from build123d import *

# Parameters (mm, degrees)
PAD_DEPTH       = 20
PAD001_DEPTH    = 10
PAD002_DEPTH    = 15
SKETCH003_R     = 2.1
POCKET_DEPTH    = 8.001
SKETCH004_R     = 3.75
POCKET001_DEPTH = 4
SKETCH005_W     = 10
SKETCH005_H     = 55
POCKET002_DEPTH = 40
SKETCH006_R     = 15
POCKET003_DEPTH = 95.001


with BuildPart() as part:
    # Sketch → Pad (new body, symmetric)
    with BuildSketch(Plane.XZ):
        Polygon((0, 163), (0, 0), (105, 0), (105, 8), (15, 8), (15, 163), align=None)
    extrude(amount=PAD_DEPTH, both=True)

    # Sketch001 (on Face8 of Pad) → Pad001 (join)
    with BuildSketch(Plane.XZ.offset(20)):
        Polygon((15, 38), (90, 8), (15, 8), align=None)
    pad001 = extrude(amount=-PAD001_DEPTH)

    # Mirrored: Pad001 across XZ
    add(pad001.mirror(Plane.XZ))

    # Sketch002 (on Face1 of Mirrored) → Pad002 (join)
    with BuildSketch(Plane(origin=(0, 0, 0), x_dir=(0, -1, 0), z_dir=(-1, 0, 0))):
        Polygon((-40, 0), (-20, 0), (-20, 163), (-30, 163), (-30, 8), (-40, 8), align=None)
    pad002 = extrude(amount=-PAD002_DEPTH)

    # Mirrored001: Pad002 across Sketch002 V_Axis
    add(pad002.mirror(Plane(origin=(0, 0, 0), x_dir=(-1, 0, 0), z_dir=(0, -1, 0))))

    # Sketch003 (on Face11 of Mirrored001) → Pocket (cut, through all)
    with BuildSketch(Plane.XY.offset(8)):
        with Locations((7.5, 35)):
            Circle(SKETCH003_R)
        with Locations((7.5, -35)):
            Circle(SKETCH003_R)
        with Locations((97, 15.5)):
            Circle(SKETCH003_R)
        with Locations((97, -15.5)):
            Circle(SKETCH003_R)
    extrude(amount=-POCKET_DEPTH, mode=Mode.SUBTRACT)

    # Sketch004 (on Face15 of Pocket) → Pocket001 (cut)
    with BuildSketch(Plane.XY.offset(8)):
        with Locations((7.5, 35)):
            Circle(SKETCH004_R)
        with Locations((97, 15.5)):
            Circle(SKETCH004_R)
        with Locations((97, -15.5)):
            Circle(SKETCH004_R)
        with Locations((7.5, -35)):
            Circle(SKETCH004_R)
    extrude(amount=-POCKET001_DEPTH, mode=Mode.SUBTRACT)

    # Sketch005 (on Face12 of Pocket001) → Pocket002 (cut)
    with BuildSketch(Plane.XZ.offset(20)):
        with Locations((5, 135.5)):
            Rectangle(SKETCH005_W, SKETCH005_H)
    extrude(amount=-POCKET002_DEPTH, mode=Mode.SUBTRACT)

    # Sketch006 (on Face23 of Pocket002) → Pocket003 (cut, through all)
    with BuildSketch(Plane(origin=(10, 0, 0), x_dir=(0, -1, 0), z_dir=(-1, 0, 0))):
        with Locations((0, 141)):
            Circle(SKETCH006_R)
    extrude(amount=-POCKET003_DEPTH, mode=Mode.SUBTRACT)


solid = part.part
Read the model definition and answer for the solid it produces. Units are mm, in the model's axes. A direction names the side the tool comes from. Round coordinates to 2 decimals unless told otherwise and drop trailing zeros. Write each loop counter-clockwise with the first axis right and the second up, starting at its lowest first coordinate (ties: lowest second). Pieces come first, ordered by that corner, then holes. Notation, with made-up numbers: (69.5, -38.5) - (112.5, -38.5) arc R29 cw to (112.5, -2.5) - close; hole circle Ø11 at (76.5, 71). An arc over 180 degrees is marked (long way). Use a Markdown table: item, result.
(1) The part is cut by section A-A (x = 7.5). Write down the section's boundary in (y, z), then the cut area to 3 significant figures.
Reported:
| item | result |
|---|---|
| outline | (-40, 0) - (-37.1, 0) - (-37.1, 4) - (-38.75, 4) - (-38.75, 8) - (-40, 8) - close; (-32.9, 0) - (32.9, 0) - (32.9, 4) - (31.25, 4) - (31.25, 8) - (30, 8) - (30, 163) - (20, 163) - (20, 108) - (-20, 108) - (-20, 163) - (-30, 163) - (-30, 8) - (-31.25, 8) - (-31.25, 4) - (-32.9, 4) - close; (37.1, 0) - (40, 0) - (40, 8) - (38.75, 8) - (38.75, 4) - (37.1, 4) - close |
| area | 7,650 mm2 |
(2) Straight lines are drawn through the part: line 1 along Y through (x, z) = (97, 2.7); line 2 along Y through (x, z) = (7.5, 2.8); line 3 along X through (y, z) = (15, 5). For each, find the intervals that lie inside material, in ascending order. Write a range as [from, to].
Reported:
| item | result |
|---|---|
| line 1 | [-20, -17.6], [-13.4, 13.4], [17.6, 20] |
| line 2 | [-40, -37.1], [-32.9, 32.9], [37.1, 40] |
| line 3 | [0, 93.28], [100.72, 105] |
(3) The part is cut by section B-B (y = 35). Write down the section's boundary in (x, z).
Reported:
| item | result |
|---|---|
| outline | (0, 0) - (5.4, 0) - (5.4, 4) - (3.75, 4) - (3.75, 8) - (0, 8) - close; (9.6, 0) - (15, 0) - (15, 8) - (11.25, 8) - (11.25, 4) - (9.6, 4) - close |
(4) Which of the six approach directions +Z, -Z, +X, -X, +Y, -Y give full straight-line access (tool end or side, diameter ignored) to faces 1 (the cylindrical face through (10.964, -36.436, 6.028)), 2 (the flat face through (7, 30, 87)), 3 (the flat face through (51, -20, 11)), 4 (the flat face through (7, -30, 87)), 5 (the flat face through (5, -20, 136))?
Reported:
| item | result |
|---|---|
| face 1 | +Z |
| face 2 | +Z, +X, -X, +Y |
| face 3 | +Z, -Z, +X, -Y |
| face 4 | +Z, +X, -X, -Y |
| face 5 | +Z, -X |
(5) The mould has two halves that part along Y. Classify faces 6 (the flat face through (7, -40, 4)), 7 (the cylindrical face through (94.9, -15.41, 2.03)), 8 (the flat face through (105, 0, 4)): released by +Y, released by -Y, zero draft, split by the parting line, or undercut.
Reported:
| item | result |
|---|---|
| face 6 | released by -Y |
| face 7 | undercut |
| face 8 | zero draft |
(6) The part is cut by section C-C (x = 97). Write down the section's boundary in (y, z).
Reported:
| item | result |
|---|---|
| outline | (-20, 0) - (-17.6, 0) - (-17.6, 4) - (-19.25, 4) - (-19.25, 8) - (-20, 8) - close; (-13.4, 0) - (13.4, 0) - (13.4, 4) - (11.75, 4) - (11.75, 8) - (-11.75, 8) - (-11.75, 4) - (-13.4, 4) - close; (17.6, 0) - (20, 0) - (20, 8) - (19.25, 8) - (19.25, 4) - (17.6, 4) - close |
(7) The part is cut by section D-D (x = 85). Write down the section's boundary in (y, z), then the cut area to 3 significant figures.
Reported:
| item | result |
|---|---|
| outline | (-20, 0) - (20, 0) - (20, 10) - (10, 10) - (10, 8) - (-10, 8) - (-10, 10) - (-20, 10) - close |
| area | 360 mm2 |
(8) Each of these flat-tipped pins is pushed along its axis until it touches: pin 1 Ø12 at (x, y) = (79.5, 7.5) entering from +Z; pin 2 Ø2 at (y, z) = (19, 43.5) entering from +X; pin 3 Ø2 at (x, y) = (8.5, -36) entering from +Z; pin 4 Ø10 at (x, y) = (30, -27) entering from -Z. Where does it stop, or does it pass through?
Reported:
| item | result |
|---|---|
| pin 1 | z = 14.38 |
| pin 2 | x = 15 |
| pin 3 | z = 4 |
| pin 4 | through |
